from build123d import *

# Parameters (mm, degrees)
BOSS_EXTRUDE1_DEPTH = 50
FILLET1_R           = 10
SKETCH2_W           = 10
SKETCH2_H           = 250
CUT_EXTRUDE4_DEPTH  = 5
SKETCH5_W           = 10
SKETCH5_H           = 5
CUT_EXTRUDE16_DEPTH = 200
SKETCH6_W           = 10
SKETCH6_H           = 5
CUT_EXTRUDE17_DEPTH = 50
FILLET2_R           = 10
FILLET3_R           = 10


with BuildPart() as part:
    # Sketch1 → Boss-Extrude1 (new body)
    with BuildSketch(Plane.XY):
        Polygon((-750, 0), (750, 0), (750, -500), (550, -500), (550, -250), (-550, -250), (-550, -500), (-750, -500), align=None)
    extrude(amount=BOSS_EXTRUDE1_DEPTH)

    # Fillet1
    fillet1_edges = [part.edges().sort_by_distance(p)[0] for p in [
        (0, -250, 0),
        (-550, -375, 0),
        (-750, -250, 0),
        (-550, -375, 50),
        (0, -250, 50),
        (550, -375, 50),
        (750, -250, 50),
        (0, 0, 50),
        (-750, -250, 50),
        (0, 0, 0),
        (750, -250, 0),
        (550, -375, 0),
    ]]
    fillet(fillet1_edges, radius=FILLET1_R)

    # Sketch2 → Cut-Extrude4 (cut)
    with BuildSketch(Plane.XY.offset(50)):
        with Locations((-545, -125)):
            Rectangle(SKETCH2_W, SKETCH2_H)
    cut_extrude4 = extrude(amount=-CUT_EXTRUDE4_DEPTH, mode=Mode.SUBTRACT)

    # Mirror1: Cut-Extrude4 across plane
    add(cut_extrude4.mirror(Plane(origin=(0, 0, 0), x_dir=(0, 0, 1), z_dir=(1, 0, 0))), mode=Mode.SUBTRACT)

    # Sketch5 → Cut-Extrude16 (cut)
    with BuildSketch(Plane(origin=(0, 0, 0), x_dir=(1, 0, 0), z_dir=(0, 1, 0))):
        with Locations((-545, -2.5)):
            Rectangle(SKETCH5_W, SKETCH5_H)
    cut_extrude16 = extrude(amount=-CUT_EXTRUDE16_DEPTH, mode=Mode.SUBTRACT)

    # Mirror5: Cut-Extrude16 across plane
    add(cut_extrude16.mirror(Plane(origin=(0, 0, 0), x_dir=(0, 0, 1), z_dir=(1, 0, 0))), mode=Mode.SUBTRACT)

    # Sketch6 → Cut-Extrude17 (cut)
    with BuildSketch(Plane.XY.offset(50)):
        with Locations((545, -2.5)):
            Rectangle(SKETCH6_W, SKETCH6_H)
    cut_extrude17 = extrude(amount=-CUT_EXTRUDE17_DEPTH, mode=Mode.SUBTRACT)

    # Fillet2
    fillet2_edges = [part.edges().sort_by_distance(p)[0] for p in [
        (545, -5, 45),
        (545, -5, 5),
    ]]
    fillet(fillet2_edges, radius=FILLET2_R)

    # Mirror8: Cut-Extrude17 across plane
    add(cut_extrude17.mirror(Plane(origin=(0, 0, 0), x_dir=(0, 0, 1), z_dir=(1, 0, 0))), mode=Mode.SUBTRACT)

    # Fillet3
    fillet3_edges = [part.edges().sort_by_distance(p)[0] for p in [
        (-545, -5, 5),
        (-545, -5, 45),
    ]]
    fillet(fillet3_edges, radius=FILLET3_R)


solid = part.part
CAD build for the part. Positions are in the model's coordinates, mm. A direction names the side the tool comes from. Round coordinates to 2 decimals unless told otherwise and drop trailing zeros. Write each loop counter-clockwise with the first axis right and the second up, starting at its lowest first coordinate (ties: lowest second). Pieces come first, ordered by that corner, then holes. Notation, with made-up numbers: M 27.25,-13.5 L 70.25,-13.5 A20 ccw 70.25,11.5 Z; hole C 43,34.5 d1. An arc over 180 degrees is marked long. Put each result on its own line as item: value. Start each with the question number.
1) Pin check, flat tips, straight feed: pin 1 Ø5 at (x, z) = (-421, 40.5) entering from -Y; pin 2 Ø8 at (x, y) = (-544.5, -87.5) entering from +Z; pin 3 Ø4 at (x, z) = (-543.5, 1.5) entering from +Y. Stop position of each tip, or through.
2) 3-axis set-ups, long thin cutter, end or side, ignore diameter. For faces 1 (the flat face through (550, -377, 25)), 2 (the flat face through (649, 0, 25)), 3 (the flat face through (540, -115.7, 45.5)): which of +Z, -Z, +X, -X, +Y, -Y reach the whole face in a straight line?
3) Pull direction X, two halves, no side cores. Call faces 4 (the flat face through (750, -247, 25)), 5 (the flat face through (-750, -253, 25)), 6 (the flat face through (8, -250, 25)): pulls with the +X half, pulls with the -X half, needs draft (parallel to the pull), parting line crosses it, or undercut.
4) Saw through at B-B, the plane x = -259.5. Write the cut outline in (y, z).
5) Drill centre lines: probe 1 along X at (y, z) = (-429, 41); probe 2 along X at (y, z) = (-382.5, 32.5); probe 3 along X at (y, z) = (-154, 46). Where is each one in solid material? Low to high. Write a range as [from, to].
6) Saw through at C-C, the plane z = 24. Write the cut outline in (x, y).
7) Saw through at A-A, the plane y = -416. Write the cut outline in (x, z).
Resolved:
1. pin 1: y = -250
1. pin 2: z = 45
1. pin 3: y = -200
2. face 1: +Z, -Z, -Y
2. face 2: +Z, -Z, +X, -X, +Y
2. face 3: +Y
3. face 4: pulls with the +X half
3. face 5: pulls with the -X half
3. face 6: undercut
4. outline: M -250,10 A10 ccw -240,0 L -10,0 A10 ccw 0,10 L 0,40 A10 ccw -10,50 L -240,50 A10 ccw -250,40 Z
5. probe 1: [-749.95, -550.05], [550.05, 749.95]
5. probe 2: [-750, -550], [550, 750]
5. probe 3: [-748, -550], [-540, 540], [550, 748]
6. outline: M -750,-500 L -550,-500 L -550,-250 L 550,-250 L 550,-500 L 750,-500 L 750,0 L 550,0 L 550,-5 L 540,-5 L 540,0 L -540,0 L -540,-5 L -550,-5 L -550,0 L -750,0 Z
7. outline: M -750,10 A10 ccw -740,0 L -560,0 A10 ccw -550,10 L -550,40 A10 ccw -560,50 L -740,50 A10 ccw -750,40 Z; M 550,10 A10 ccw 560,0 L 740,0 A10 ccw 750,10 L 750,40 A10 ccw 740,50 L 560,50 A10 ccw 550,40 Z
